Work out the finished part from the listing and answer in its coordinate system (mm). A direction names the side the tool comes from. Give positions to 0.01 mm unless a question says otherwise; leave off trailing zeros. Loops run counter-clockwise (first coordinate to the right, second up) from the corner with the lowest first, then second, coordinate; pieces in that order, holes last. Notation, with made-up numbers: (74, 48.5) - (79, 48.5) arc R30 ccw to (79, 85.5) - close; hole circle Ø4 at (59, 40.25). An arc over 180 degrees is marked (long way). Use one line per item in the form item = value. Start each with the question number.
from build123d import *

# Parameters (mm, degrees)
BOSS_EXTRUDE1_DEPTH = 1.6002
SKETCH3_R           = 1.1049
SKETCH3_R_2         = 1.651
SKETCH3_R_3         = 1.5875
SKETCH3_R_4         = 0.4826
CUT_EXTRUDE1_DEPTH  = 2.6002
SKETCH4_R           = 0.508
SKETCH4_R_2         = 0.4064
CUT_EXTRUDE2_DEPTH  = 2.6002


with BuildPart() as part:
    # Sketch2 → Boss-Extrude1 (new body)
    with BuildSketch(Plane.XY):
        Polygon((-34.2899492, 26.67), (30.2259492, 26.67), (31.7499492, 25.146), (31.7499492, 13.716), (34.2899492, 11.176), (34.2899492, -21.59), (31.7499492, -24.13), (31.7499492, -26.67), (-34.2899492, -26.67), align=None)
    extrude(amount=-BOSS_EXTRUDE1_DEPTH)

    # Sketch3 → Cut-Extrude1 (cut, through all)
    with BuildSketch(Plane.XY):
        with Locations((-30.4799492, 17.429988)):
            Circle(SKETCH3_R)
        with Locations((-30.4799492, 5.430012)):
            Circle(SKETCH3_R)
        with Locations((-28.6003492, -18.3642)):
            Circle(SKETCH3_R_2)
        with Locations((-25.6031492, -23.368)):
            Circle(SKETCH3_R_2)
        with Locations((-22.6060508, -18.3642)):
            Circle(SKETCH3_R_2)
        with Locations((31.7499492, -19.05)):
            Circle(SKETCH3_R_3)
        with Locations((31.7499492, 8.89)):
            Circle(SKETCH3_R_3)
        with Locations((-19.0500508, 24.13)):
            Circle(SKETCH3_R_3)
        with Locations((-25.769951, 12.679934)):
            Circle(SKETCH3_R_4)
        with Locations((-27.769947, 12.679934)):
            Circle(SKETCH3_R_4)
        with Locations((-27.769947, 10.180066)):
            Circle(SKETCH3_R_4)
        with Locations((-25.769951, 10.180066)):
            Circle(SKETCH3_R_4)
        with Locations((-20.3200508, -24.13)):
            Circle(SKETCH3_R_3)
    extrude(amount=-CUT_EXTRUDE1_DEPTH, mode=Mode.SUBTRACT)

    # Sketch4 → Cut-Extrude2 (cut, through all)
    with BuildSketch(Plane.XY):
        with Locations((29.2099492, 24.13)):
            Circle(SKETCH4_R)
        with Locations((26.6699492, 24.13)):
            Circle(SKETCH4_R)
        with Locations((24.1299492, 24.13)):
            Circle(SKETCH4_R)
        with Locations((21.5899492, 24.13)):
            Circle(SKETCH4_R)
        with Locations((19.0499492, 24.13)):
            Circle(SKETCH4_R)
        with Locations((16.5099492, 24.13)):
            Circle(SKETCH4_R)
        with Locations((13.9699492, 24.13)):
            Circle(SKETCH4_R)
        with Locations((11.4299492, 24.13)):
            Circle(SKETCH4_R)
        with Locations((7.3659492, 24.13)):
            Circle(SKETCH4_R)
        with Locations((4.8259492, 24.13)):
            Circle(SKETCH4_R)
        with Locations((2.2859492, 24.13)):
            Circle(SKETCH4_R)
        with Locations((-0.2540508, 24.13)):
            Circle(SKETCH4_R)
        with Locations((-2.7940508, 24.13)):
            Circle(SKETCH4_R)
        with Locations((-5.3340508, 24.13)):
            Circle(SKETCH4_R)
        with Locations((-7.8740508, 24.13)):
            Circle(SKETCH4_R)
        with Locations((-10.4140508, 24.13)):
            Circle(SKETCH4_R)
        with Locations((28.5749492, -6.477)):
            Circle(SKETCH4_R_2)
        with Locations((26.0349492, -6.477)):
            Circle(SKETCH4_R_2)
        with Locations((23.4949492, -6.477)):
            Circle(SKETCH4_R_2)
        with Locations((20.9549492, -6.477)):
            Circle(SKETCH4_R_2)
        with Locations((18.4149492, -6.477)):
            Circle(SKETCH4_R_2)
        with Locations((15.8749492, -6.477)):
            Circle(SKETCH4_R_2)
        with Locations((13.3349492, -6.477)):
            Circle(SKETCH4_R_2)
        with Locations((10.7949492, -6.477)):
            Circle(SKETCH4_R_2)
        with Locations((8.2549492, -6.477)):
            Circle(SKETCH4_R_2)
        with Locations((5.7149492, -6.477)):
            Circle(SKETCH4_R_2)
        with Locations((3.1749492, -6.477)):
            Circle(SKETCH4_R_2)
        with Locations((0.6349492, -6.477)):
            Circle(SKETCH4_R_2)
        with Locations((-1.9050508, -6.477)):
            Circle(SKETCH4_R_2)
        with Locations((-4.4450508, -6.477)):
            Circle(SKETCH4_R_2)
        with Locations((28.5749492, -14.097)):
            Circle(SKETCH4_R_2)
        with Locations((26.0349492, -14.097)):
            Circle(SKETCH4_R_2)
        with Locations((23.4949492, -14.097)):
            Circle(SKETCH4_R_2)
        with Locations((20.9549492, -14.097)):
            Circle(SKETCH4_R_2)
        with Locations((18.4149492, -14.097)):
            Circle(SKETCH4_R_2)
        with Locations((15.8749492, -14.097)):
            Circle(SKETCH4_R_2)
        with Locations((13.3349492, -14.097)):
            Circle(SKETCH4_R_2)
        with Locations((10.7949492, -14.097)):
            Circle(SKETCH4_R_2)
        with Locations((8.2549492, -14.097)):
            Circle(SKETCH4_R_2)
        with Locations((5.7149492, -14.097)):
            Circle(SKETCH4_R_2)
        with Locations((3.1749492, -14.097)):
            Circle(SKETCH4_R_2)
        with Locations((0.6349492, -14.097)):
            Circle(SKETCH4_R_2)
        with Locations((-1.9050508, -14.097)):
            Circle(SKETCH4_R_2)
        with Locations((-4.4450508, -14.097)):
            Circle(SKETCH4_R_2)
        with Locations((29.2099492, -24.13)):
            Circle(SKETCH4_R)
        with Locations((11.4299492, -24.13)):
            Circle(SKETCH4_R)
        with Locations((26.6699492, -24.13)):
            Circle(SKETCH4_R)
        with Locations((8.8899492, -24.13)):
            Circle(SKETCH4_R)
        with Locations((24.1299492, -24.13)):
            Circle(SKETCH4_R)
        with Locations((6.3499492, -24.13)):
            Circle(SKETCH4_R)
        with Locations((21.5899492, -24.13)):
            Circle(SKETCH4_R)
        with Locations((3.8099492, -24.13)):
            Circle(SKETCH4_R)
        with Locations((19.0499492, -24.13)):
            Circle(SKETCH4_R)
        with Locations((1.2699492, -24.13)):
            Circle(SKETCH4_R)
        with Locations((16.5099492, -24.13)):
            Circle(SKETCH4_R)
        with Locations((-1.2700508, -24.13)):
            Circle(SKETCH4_R)
        with Locations((-13.4620508, 20.828)):
            Circle(SKETCH4_R)
        with Locations((-13.4620508, 18.288)):
            Circle(SKETCH4_R)
        with Locations((-16.0020508, 18.288)):
            Circle(SKETCH4_R)
        with Locations((-16.0020508, 20.828)):
            Circle(SKETCH4_R)
        with Locations((-18.5420508, 18.288)):
            Circle(SKETCH4_R)
        with Locations((-18.5420508, 20.828)):
            Circle(SKETCH4_R)
        with Locations((31.8901572, -1.320038)):
            Circle(SKETCH4_R)
        with Locations((29.3501572, -1.320038)):
            Circle(SKETCH4_R)
        with Locations((29.3501572, 1.219962)):
            Circle(SKETCH4_R)
        with Locations((31.8901572, 1.219962)):
            Circle(SKETCH4_R)
        with Locations((29.3501572, 3.759962)):
            Circle(SKETCH4_R)
        with Locations((31.8901572, 3.759962)):
            Circle(SKETCH4_R)
    extrude(amount=-CUT_EXTRUDE2_DEPTH, mode=Mode.SUBTRACT)


solid = part.part
1) Determine the mould class of faces 1 (the flat face through (33.002, 12.464, -0.789)), 2 (the flat face through (-1, -26.67, -1)), 3 (the flat face through (34.29, -5, -1)), 4 (the cylindrical face through (-23.916, -19.369, -0.789)) for opening direction Y: released by +Y, released by -Y, zero draft, split by the parting line, or undercut.
2) A cutting plane is placed at B-B (y = 15). Give the vertices of the cut face in (x, z).
3) A tool of negligible diameter and unlimited length cuts with its end or side. For faces 5 (the flat face through (31.75, -25, -1)), 6 (the flat face through (31.75, 20, -1)), 7 (the flat face through (-2, 26.67, -1)), from which of +Z, -Z, +X, -X, +Y, -Y can it reach the whole face along a straight path? Write none if from no direction.
4) Find the intervals of material crossed by probe 1 along Y at (x, z) = (24, -0.4); probe 2 along Y at (x, z) = (23.5, -1); probe 3 along Y at (x, z) = (14, -1.1), in increasing order.
5) A flat-ended cylindrical pin translates along its axis: pin 1 Ø0.5 at (y, z) = (20, -0.5) entering from +X. Find the tip coordinate at first contact, or state that the pin passes through.
6) A cutting plane is placed at C-C (z = -0.75). State how many separate pieces and enclosed holes the cut face has, plus the area to 3 significant figures.
7) A cutting plane is placed at A-A (y = 8.89). Give the vertices of the cut face in (x, z).
Answer sheet:
q1.face_1 = released by +Y
q1.face_2 = released by -Y
q1.face_3 = zero draft
q1.face_4 = undercut
q2.outline = (-34.29, -1.6) - (31.75, -1.6) - (31.75, 0) - (-34.29, 0) - close
q3.face_5 = +Z, -Z, +X, -Y
q3.face_6 = +Z, -Z, +X, +Y
q3.face_7 = +Z, -Z, +X, -X, +Y
q4.probe_1 = -26.67 to -24.62, -23.64 to 23.64, 24.62 to 26.67
q4.probe_2 = -26.67 to -14.5, -13.69 to -6.88, -6.07 to 26.67
q4.probe_3 = -26.67 to 23.62, 24.64 to 26.67
q5.pin_1 = 31.75
q6.separate_pieces = 1
q6.enclosed_holes = 81
q6.area = 3,500 mm²
q7.outline = (-34.29, -1.6) - (30.16, -1.6) - (30.16, 0) - (-34.29, 0) - close; (33.34, -1.6) - (34.29, -1.6) - (34.29, 0) - (33.34, 0) - close
